```python
from build123d import *

# Parameters (mm, degrees)
SALIENTE_EXTRUIR1_DEPTH = 3


with BuildPart() as part:
    # Croquis1 → Saliente-Extruir1 (new body)
    with BuildSketch(Plane.XY):
        with BuildLine():
            Line((-0.6, -15.075), (0.6, -15.075))
            ThreePointArc((0.6, -15.075), (10.853048327, -10.828048327), (15.1, -0.575))
            Line((15.1, -0.575), (15.1, 0.575))
            ThreePointArc((15.1, 0.575), (10.853048327, 10.828048327), (0.6, 15.075))
            Line((0.6, 15.075), (-0.6, 15.075))
            ThreePointArc((-0.6, 15.075), (-10.853048327, 10.828048327), (-15.1, 0.575))
            Line((-15.1, 0.575), (-15.1, -0.575))
            ThreePointArc((-15.1, -0.575), (-10.853048327, -10.828048327), (-0.6, -15.075))
        make_face()
        Polygon((-12.6, -2.5), (-12.6, 0.5), (-1.5, 0.5), (-1.5, 12.575), (1.5, 12.575), (1.5, 0.5), (12.6, 0.5), (12.6, -2.5), (1.5, -2.5), (1.5, -12.575), (-1.5, -12.575), (-1.5, -2.5), align=None, mode=Mode.SUBTRACT)
    extrude(amount=SALIENTE_EXTRUIR1_DEPTH)


solid = part.part
```
Can you work these out from the model? Positions are in its coordinate system, mm. A direction names the side the tool comes from. Coordinates: 2 decimals unless noted, no trailing zeros. Loops run counter-clockwise (first coordinate to the right, second up) from the corner with the lowest first, then second, coordinate; pieces in that order, holes last.
1) Which directions (+Z, -Z, +X, -X, +Y, -Y) give clear straight access to the entire face, cutting with the end or side of a thin tool? Please do faces 1 (the cylindrical face through (10.74, -10.94, 1.48)), 2 (the flat face through (-7, 0.5, 1)).
2) For pin 1 (1.5 mm diameter, centred on y = 4, z = 2, fed in from -X); pin 2 (1.5 mm diameter, centred on x = 9, z = 1.5, fed in from -Y); pin 3 (1.5 mm diameter, centred on x = 6, z = 1, fed in from +Y), each with a flat end and sliding along its axis, tell me the tip position at first contact or that it passes through.
3) Imagine slicing it at A-A on z = 2.4. List the corners of the cut face in (x, y) for me (3 decimals), plus the area to 3 significant figures.
4) Thinking about a two-plate mould opening in Y: for faces 3 (the flat face through (0, -15.075, 1)), 4 (the flat face through (-1.5, 6, 1)), 5 (the flat face through (-15.1, 0, 1)), 6 (the flat face through (7, -2.5, 1)), which applies, pulls with the +Y half, pulls with the -Y half, needs draft (parallel to the pull), parting line crosses it, or undercut?
5) I need wall thicknesses on probe 1 along Y at (x, z) = (-1, 0.25) (3 decimals); probe 2 along X at (y, z) = (-6, 0.2); probe 3 along Y at (x, z) = (11.5, 0.3). Which ranges of each line are inside material? Lowest first, please.
6) Imagine slicing it at C-C on x = -10. List the corners of the cut face in (y, z) for me, plus the area to 3 significant figures.
7) Imagine slicing it at B-B on y = -2. List the corners of the cut face in (x, z) for me.
Completed:
1. face 1: +Z, -Z, +X, -Y
1. face 2: +Z, -Z
2. pin 1: stops at x = -14.85
2. pin 2: stops at y = -12.89
2. pin 3: stops at y = 14.31
3. outline: (-15.1, -0.575) arc R14.5 ccw to (-0.6, -15.075) - (0.6, -15.075) arc R14.5 ccw to (15.1, -0.575) - (15.1, 0.575) arc R14.5 ccw to (0.6, 15.075) - (-0.6, 15.075) arc R14.5 ccw to (-15.1, 0.575) - close; hole (-12.6, -2.5) - (-1.5, -2.5) - (-1.5, -12.575) - (1.5, -12.575) - (1.5, -2.5) - (12.6, -2.5) - (12.6, 0.5) - (1.5, 0.5) - (1.5, 12.575) - (-1.5, 12.575) - (-1.5, 0.5) - (-12.6, 0.5) - close
3. area: 588 mm2
4. face 3: pulls with the -Y half
4. face 4: undercut
4. face 5: needs draft
4. face 6: undercut
5. probe 1: y = -15.069 to -12.575, 12.575 to 15.069
5. probe 2: x = -14.05 to -1.5, 1.5 to 14.05
5. probe 3: y = -10.14 to -2.5, 0.5 to 10.14
6. outline: (-11.62, 0) - (-2.5, 0) - (-2.5, 3) - (-11.62, 3) - close; (0.5, 0) - (11.62, 0) - (11.62, 3) - (0.5, 3) - close
6. area: 60.7 mm2
7. outline: (-15.03, 0) - (-12.6, 0) - (-12.6, 3) - (-15.03, 3) - close; (12.6, 0) - (15.03, 0) - (15.03, 3) - (12.6, 3) - close
